Design review of the part shown in the three views and the two pictorial views. Dimensions are in mm from the part's minimum x, y and z. Give positions to 0.01 mm unless a question says otherwise; leave off trailing zeros. Loops run counter-clockwise (first coordinate to the right, second up) from the corner with the lowest first, then second, coordinate; pieces in that order, holes last. Notation, with made-up numbers: (43, 70.5) -> (91, 70.5) arc R13 cw to (91, 77.5) -> close; hole circle Ø3 at (65, 21). An arc over 180 degrees is marked (long way). Use CSV: the item, a comma, the result in double quotes. Start each with the question number.
Item 1: We need section C-C (x = 61). State the section outline as (y, z) points, plus the area to 3 significant figures.
Item 2: We need section B-B (x = 5). State the section outline as (y, z) points, plus the area to 3 significant figures.
Item 3: We need section A-A (z = 5). State the section outline as (x, y) points, plus the area to 3 significant figures.
Item 4: Wall thickness on line 1 along X through (y, z) = (0.45, 5); line 2 along Z through (x, y) = (48, 8.5): over which ranges is each line inside the solid? List them lowest first. Write a range as from..to.
Item 5: We need section D-D (x = 30.5). State the section outline as (y, z) points, plus the area to 3 significant figures.
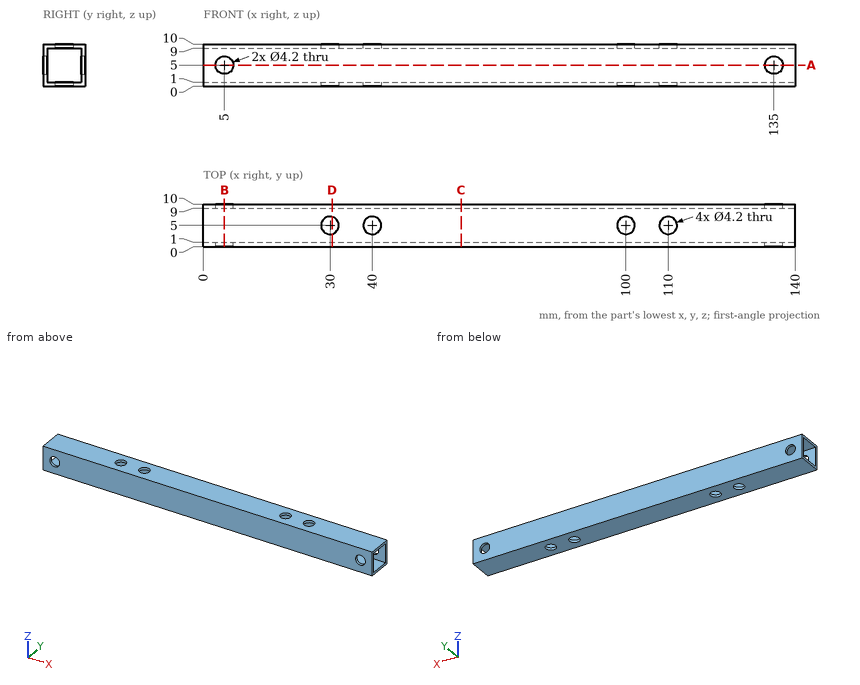
Results found:
1,outline,"(0, 0) -> (10, 0) -> (10, 10) -> (0, 10) -> close; hole (1, 1) -> (9, 1) -> (9, 9) -> (1, 9) -> close"
1,area,"36.0 mm²"
2,outline,"(0, 0) -> (10, 0) -> (10, 2.9) -> (9, 2.9) -> (9, 1) -> (1, 1) -> (1, 2.9) -> (0, 2.9) -> close; (0, 7.1) -> (1, 7.1) -> (1, 9) -> (9, 9) -> (9, 7.1) -> (10, 7.1) -> (10, 10) -> (0, 10) -> close"
2,area,"27.6 mm²"
3,outline,"(0, 0) -> (2.9, 0) -> (2.9, 1) -> (0, 1) -> close; (0, 9) -> (2.9, 9) -> (2.9, 10) -> (0, 10) -> close; (7.1, 0) -> (132.9, 0) -> (132.9, 1) -> (7.1, 1) -> close; (7.1, 9) -> (132.9, 9) -> (132.9, 10) -> (7.1, 10) -> close; (137.1, 0) -> (140, 0) -> (140, 1) -> (137.1, 1) -> close; (137.1, 9) -> (140, 9) -> (140, 10) -> (137.1, 10) -> close"
3,area,"263 mm²"
4,line 1,"0..2.9, 7.1..132.9, 137.1..140"
4,line 2,"0..1, 9..10"
5,outline,"(0, 0) -> (2.96, 0) -> (2.96, 1) -> (1, 1) -> (1, 9) -> (2.96, 9) -> (2.96, 10) -> (0, 10) -> close; (7.04, 0) -> (10, 0) -> (10, 10) -> (7.04, 10) -> (7.04, 9) -> (9, 9) -> (9, 1) -> (7.04, 1) -> close"
5,area,"27.8 mm²"
